The model under review builds one solid part; all positions refer to its coordinate system, in mm. Face numbers are marked on the shaded views. Give positions to 0.01 mm unless a question says otherwise; leave off trailing zeros. Order: outer loops, then holes, each group sorted by start corner. A loop starts at its lowest first (then second) coordinate and runs counter-clockwise, first axis right, second up. Notation, with made-up numbers: (28, 23.5) - (76, 23.5) arc R17 cw to (76, 52.5) - close; hole circle Ø7 at (33, 48.5). An arc over 180 degrees is marked (long way). Write item = value, one per line. Start each with the question number.
1. Mouldability with a two-part tool opening along Y and no side actions: class the marked faces 1, 2, 3 and 4 as pulls with the +Y half, pulls with the -Y half, needs draft (parallel to the pull), parting line crosses it, or undercut.
2. We need section B-B, the plane y = -9. Give the boundary of the cut face in (x, z) (1 decimal).
3. We need section D-D, the plane y = 0. Give the boundary of the cut face in (x, z) (3 decimals), and give its area (3 significant figures).
4. Wall thickness on probe 1 along Z at (x, y) = (9, 11) (3 decimals); probe 2 along X at (y, z) = (-0.5, 4); probe 3 along X at (y, z) = (11.5, 6): over which ranges is each line inside the solid? List them lowest first.
5. We need section A-A, the plane x = 0. Give the boundary of the cut face in (y, z) (3 decimals), and give its area (3 significant figures).
6. We need section C-C, the plane z = 1.75. Give the boundary of the cut face in (x, y) (1 decimal), and give its area (3 significant figures).
7. For P1, Ø3, axis at x = -26.65, z = 4.76, coming from the -Y side (3 decimals); P2, Ø0.9, axis at x = 38.5, z = 4.5, coming from the +Y side (3 decimals); P3, Ø2, axis at x = 26.69, z = 4.76, coming from the +Y side; P4, Ø2.5, axis at x = 26.69, z = 4.76, coming from the -Y side, all flat-tipped, find the tip position at first contact; note any pin that passes through.
from build123d import *

# Parameters (mm, degrees)
SKETCH1_R           = 1.7
SKETCH1_R_2         = 7
BOSS_EXTRUDE1_DEPTH = 9.525
LPATTERN1_COUNT     = 4
LPATTERN1_PITCH     = 17.78
SKETCH13_R          = 1.4732
CUT_EXTRUDE1_DEPTH  = 12.7


with BuildPart() as part:
    # Sketch1 → Boss-Extrude1 (new body)
    with BuildSketch(Plane.XY):
        Polygon((-44.432958233, 15.875), (44.467041767, 15.875), (44.467041767, -15.875), (-44.432958233, -15.875), (-53.519229126, -13.0175), align=None)
        with Locations((0, -9)):
            Circle(SKETCH1_R, mode=Mode.SUBTRACT)
        with Locations((-9, 0)):
            Circle(SKETCH1_R, mode=Mode.SUBTRACT)
        with Locations((0, 9)):
            Circle(SKETCH1_R, mode=Mode.SUBTRACT)
        with Locations((9, 0)):
            Circle(SKETCH1_R, mode=Mode.SUBTRACT)
        Circle(SKETCH1_R_2, mode=Mode.SUBTRACT)
    extrude(amount=BOSS_EXTRUDE1_DEPTH)

    # Sketch12 → Tap Drill for #6-32 Tap1 (revolve, cut)
    with BuildSketch(Plane(origin=(26.687041767, -15.875, 4.7625), x_dir=(0, 0, -1), z_dir=(1, 0, 0))):
        Polygon((0, 0), (0, 13.51269403), (1.35255, 12.7), (1.35255, 0), align=None)
    tap_drill_for_6_32_tap1 = revolve(axis=Axis((26.687041767, -22.225, 4.7625), (0, 1, 0)), mode=Mode.SUBTRACT)

    # LPattern1: Tap Drill for #6-32 Tap1 ×4
    with Locations(*[(-i * LPATTERN1_PITCH, 0, 0) for i in range(1, LPATTERN1_COUNT)]):
        add(tap_drill_for_6_32_tap1, mode=Mode.SUBTRACT)

    # Mirror8: Tap Drill for #6-32 Tap1 across plane
    add(tap_drill_for_6_32_tap1.mirror(Plane.ZX), mode=Mode.SUBTRACT)

    # Mirror8 copy 1 sketch → Mirror8 copy 1 (revolve, cut)
    with BuildSketch(Plane(origin=(8.907041767, 15.875, 4.7625), x_dir=(0, 0, -1), z_dir=(1, 0, 0))):
        Polygon((0, 0), (0, -13.51269403), (1.35255, -12.7), (1.35255, 0), align=None)
    revolve(axis=Axis((8.907041767, 22.225, 4.7625), (0, 1, 0)), mode=Mode.SUBTRACT)

    # Mirror8 copy 2 sketch → Mirror8 copy 2 (revolve, cut)
    with BuildSketch(Plane(origin=(-8.872958233, 15.875, 4.7625), x_dir=(0, 0, -1), z_dir=(1, 0, 0))):
        Polygon((0, 0), (0, -13.51269403), (1.35255, -12.7), (1.35255, 0), align=None)
    revolve(axis=Axis((-8.872958233, 22.225, 4.7625), (0, 1, 0)), mode=Mode.SUBTRACT)

    # Mirror8 copy 3 sketch → Mirror8 copy 3 (revolve, cut)
    with BuildSketch(Plane(origin=(-26.652958233, 15.875, 4.7625), x_dir=(0, 0, -1), z_dir=(1, 0, 0))):
        Polygon((0, 0), (0, -13.51269403), (1.35255, -12.7), (1.35255, 0), align=None)
    revolve(axis=Axis((-26.652958233, 22.225, 4.7625), (0, 1, 0)), mode=Mode.SUBTRACT)

    # Sketch13 → Cut-Extrude1 (cut)
    with BuildSketch(Plane.XZ.offset(15.875)):
        with Locations((38.117041767, 4.7625)):
            Circle(SKETCH13_R)
    cut_extrude1 = extrude(amount=-CUT_EXTRUDE1_DEPTH, mode=Mode.SUBTRACT)

    # Mirror9: Cut-Extrude1 across plane
    add(cut_extrude1.mirror(Plane.ZX), mode=Mode.SUBTRACT)


solid = part.part
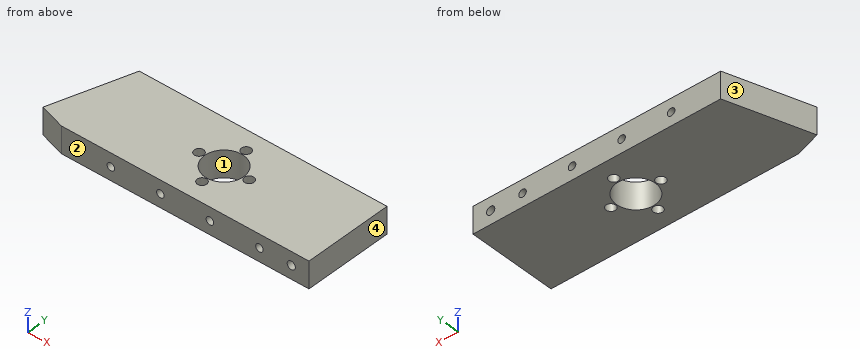
Model answer:
q1.face_1 = undercut
q1.face_2 = pulls with the -Y half
q1.face_3 = pulls with the +Y half
q1.face_4 = needs draft
q2.outline = (-52.3, 0) - (-1.7, 0) - (-1.7, 9.5) - (-52.3, 9.5) - close; (1.7, 0) - (44.5, 0) - (44.5, 9.5) - (1.7, 9.5) - close; hole circle Ø2.7 at (-26.7, 4.8); hole circle Ø2.7 at (-8.9, 4.8); hole circle Ø2.7 at (8.9, 4.8); hole circle Ø2.7 at (26.7, 4.8); hole circle Ø2.9 at (38.1, 4.8)
q3.outline = (-49.425, 0) - (-10.7, 0) - (-10.7, 9.525) - (-49.425, 9.525) - close; (-7.3, 0) - (-7, 0) - (-7, 9.525) - (-7.3, 9.525) - close; (7, 0) - (7.3, 0) - (7.3, 9.525) - (7, 9.525) - close; (10.7, 0) - (44.467, 0) - (44.467, 9.525) - (10.7, 9.525) - close
q3.area = 696 mm2
q4.probe_1 = 0 to 3.413, 6.112 to 9.525
q4.probe_2 = -49.58 to -10.62, -7.38 to -6.98, 6.98 to 7.38, 10.62 to 44.47
q4.probe_3 = -45.81 to -27.2, -26.11 to -9.42, -8.33 to 8.36, 9.45 to 26.14, 27.23 to 37.32, 38.92 to 44.47
q5.outline = (-15.875, 0) - (-10.7, 0) - (-10.7, 9.525) - (-15.875, 9.525) - close; (-7.3, 0) - (-7, 0) - (-7, 9.525) - (-7.3, 9.525) - close; (7, 0) - (7.3, 0) - (7.3, 9.525) - (7, 9.525) - close; (10.7, 0) - (15.875, 0) - (15.875, 9.525) - (10.7, 9.525) - close
q5.area = 104 mm2
q6.outline = (-53.5, -13) - (-44.4, -15.9) - (44.5, -15.9) - (44.5, 15.9) - (-44.4, 15.9) - close; hole circle Ø3.4 at (-9, 0); hole circle Ø14 at (0, 0); hole circle Ø3.4 at (0, -9); hole circle Ø3.4 at (0, 9); hole circle Ø3.4 at (9, 0)
q6.area = 2,780 mm2
q7.P1 = -15.875
q7.P2 = 3.175
q7.P3 = 2.97
q7.P4 = -3.12
